Verification items for the finished model (mm, model axes). Face numbers are marked on the shaded views. A direction names the side the tool comes from. Round coordinates to 2 decimals unless told otherwise and drop trailing zeros. Order: outer loops, then holes, each group sorted by start corner. A loop starts at its lowest first (then second) coordinate and runs counter-clockwise, first axis right, second up. Notation, with made-up numbers: M 5,41.25 L 31,41.25 A37 cw 31,78.25 Z; hole C -1.75,57.5 d6. An arc over 180 degrees is marked long. Use CSV: the item, a comma, the result in double quotes. Start each with the question number.
Q1. Mould release check, pull along X, two halves, no side actions. Record for the marked faces 4, 5 and 6: +X half, -X half, draft (parallel to the pull), parting line (faces both ways), or undercut.
Q2. Sectioned sample at C-C (y = 43). Enter the section's corners in (x, z).
Q3. Gauge pin test, flat ends, axial feed: pin 1 Ø8 at (y, z) = (-23.5, 9) entering from +X; pin 2 Ø9.5 at (y, z) = (-44.5, 5) entering from -X (3 decimals); pin 3 Ø8 at (x, y) = (22, 40.5) entering from +Z; pin 4 Ø12 at (y, z) = (19, 25.5) entering from +X. Record the tip position at first contact, or that the pin passes through.
Q4. Scan lines: line 1 (Z direction, x = -14, y = 22.5); line 2 (Y direction, x = 12, z = 33.5); line 3 (X direction, y = -28.5, z = 9). Record each from-to range of solid material in increasing order.
Q5. Sectioned sample at D-D (x = -22). Enter the section's corners in (y, z), and give its area (3 significant figures).
Q6. Set-up check for the marked faces 1, 2 and 3: record each of +Z, -Z, +X, -X, +Y, -Y from which the full face is reachable in a straight line by a thin tool's end or side.
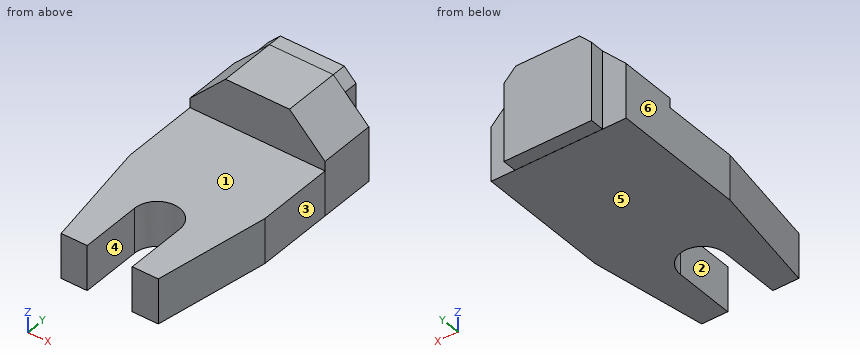
```python
from build123d import *

# Parameters (mm, degrees)
SKETCH2_W           = 57
SKETCH2_H           = 105
BOSS_EXTRUDE1_DEPTH = 19
CUT_EXTRUDE1_DEPTH  = 19
CUT_EXTRUDE2_DEPTH  = 19
CUT_EXTRUDE3_DEPTH  = 63.685724053
BOSS_EXTRUDE2_DEPTH = 24
BOSS_EXTRUDE3_DEPTH = 6


with BuildPart() as part:
    # Sketch2 → Boss-Extrude1 (new body)
    with BuildSketch(Plane.XY):
        Rectangle(SKETCH2_W, SKETCH2_H)
    extrude(amount=BOSS_EXTRUDE1_DEPTH)

    # Sketch5 → Cut-Extrude1 (cut)
    with BuildSketch(Plane.XY.offset(19)):
        Polygon((28.5, -52.5), (20.5, -52.5), (28.5, -4.5), align=None)
    extrude(amount=-CUT_EXTRUDE1_DEPTH, mode=Mode.SUBTRACT)

    # Sketch6 → Cut-Extrude2 (cut)
    with BuildSketch(Plane.XY.offset(19)):
        Polygon((-28.5, -52.5), (-28.5, -4.5), (-20.5, -52.5), align=None)
    extrude(amount=-CUT_EXTRUDE2_DEPTH, mode=Mode.SUBTRACT)

    # Sketch7 → Cut-Extrude3 (cut, through all)
    with BuildSketch(Plane.XY.offset(19)):
        with BuildLine():
            Line((-9.5, -52.5), (-9.5, -26.5))
            ThreePointArc((-9.5, -26.5), (0, -17), (9.5, -26.5))
            Line((9.5, -26.5), (9.5, -52.5))
            Line((9.5, -52.5), (-9.5, -52.5))
        make_face()
    extrude(amount=-CUT_EXTRUDE3_DEPTH, mode=Mode.SUBTRACT)

    # Sketch9 → Boss-Extrude2 (add)
    with BuildSketch(Plane(origin=(0, 52.5, 0), x_dir=(1, 0, 0), z_dir=(0, 1, 0))):
        Polygon((-28.5, -23), (-13.5, -38), (13.501670398, -38), (28.501670398, -23), (28.501670398, 0), (-28.5, 0), align=None)
    extrude(amount=-BOSS_EXTRUDE2_DEPTH)

    # Sketch10 → Boss-Extrude3 (add)
    with BuildSketch(Plane(origin=(0, 52.5, 0), x_dir=(1, 0, 0), z_dir=(0, 1, 0))):
        Polygon((18.5, -0.029901303), (-18.5, -0.029901303), (-18.5, -32.973175132), (-13.5, -37.973175132), (13.5, -37.973175132), (18.5, -32.973175132), align=None)
    extrude(amount=BOSS_EXTRUDE3_DEPTH)


solid = part.part
```
Verdict:
1,face 4,"undercut"
1,face 5,"draft"
1,face 6,"-X half"
2,outline,"M -28.5,0 L 28.5,0 L 28.5,23 L 13.5,38 L -13.5,38 L -28.5,23 Z"
3,pin 1,"stops at x = 26"
3,pin 2,"stops at x = -22.625"
3,pin 3,"stops at z = 33.5"
3,pin 4,"passes through"
4,line 1,"z = 0 to 19"
4,line 2,"y = 28.5 to 58.5"
4,line 3,"x = -24.5 to -9.5, 9.5 to 24.5"
5,outline,"M -43.5,0 L 52.5,0 L 52.5,29.5 L 28.5,29.5 L 28.5,19 L -43.5,19 Z"
5,area,"2,080 mm²"
6,face 1,"+Z, +X, -X, -Y"
6,face 2,"+Z, -Z, -Y"
6,face 3,"+Z, -Z, +X, +Y, -Y"
